Input: part model. Units: mm. Frame: model coordinates. Face numbers are marked on the shaded views. Coordinates: 2 decimals unless noted, no trailing zeros. Order: outer loops, then holes, each group sorted by start corner. A loop starts at its lowest first (then second) coordinate and runs counter-clockwise, first axis right, second up. Notation, with made-up numbers: M 51.25,80.25 L 83.25,80.25 A17 ccw 83.25,106.25 Z; hole C -39.5,-13 d3. An arc over 180 degrees is marked long. One line per item, written item: value.
```python
from build123d import *

# Parameters (mm, degrees)
SKETCH1_W           = 23.075946232
SKETCH1_H           = 15.72
SKETCH1_R           = 1.525
SKETCH1_R_2         = 4.5
BOSS_EXTRUDE2_DEPTH = 4


with BuildPart() as part:
    # Sketch1 → Boss-Extrude2 (new body)
    with BuildSketch(Plane.XY):
        Rectangle(SKETCH1_W, SKETCH1_H)
        with Locations((-8.105997779, -4.68)):
            Circle(SKETCH1_R, mode=Mode.SUBTRACT)
        with Locations((8.105997779, -4.68)):
            Circle(SKETCH1_R, mode=Mode.SUBTRACT)
        with Locations((8.105997779, 4.68)):
            Circle(SKETCH1_R, mode=Mode.SUBTRACT)
        with Locations((-8.105997779, 4.68)):
            Circle(SKETCH1_R, mode=Mode.SUBTRACT)
        Polygon((3.671947712, -6.36), (7.343895424, 0), (3.671947712, 6.36), (-3.671947712, 6.36), (-7.343895424, 0), (-3.671947712, -6.36), align=None, mode=Mode.SUBTRACT)
        Polygon((-3.671947712, -6.36), (3.671947712, -6.36), (7.343895424, 0), (3.671947712, 6.36), (-3.671947712, 6.36), (-7.343895424, 0), align=None)
        Circle(SKETCH1_R_2, mode=Mode.SUBTRACT)
    extrude(amount=BOSS_EXTRUDE2_DEPTH)


solid = part.part
```
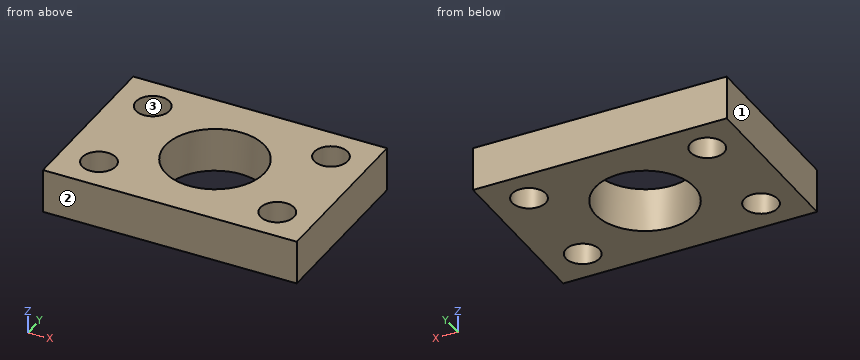
(1) Cut plane C-C on y = 0. Output: boundary loops of the cut face in (x, z).
Data:
outline: M -11.54,0 L -4.5,0 L -4.5,4 L -11.54,4 Z; M 4.5,0 L 11.54,0 L 11.54,4 L 4.5,4 Z
(2) Cut plane A-A on x = 0. Output: boundary loops of the cut face in (y, z).
Data:
outline: M -7.86,0 L -4.5,0 L -4.5,4 L -7.86,4 Z; M 4.5,0 L 7.86,0 L 7.86,4 L 4.5,4 Z
(3) Ray query, line 1 (Y direction, x = -8, z = 0.75); line 2 (X direction, y = 5, z = 0.2); line 3 (Y direction, x = -3.25, z = 3.05). Return the intervals inside material, ascending. Write a range as from..to.
Data:
line 1: y = -7.86..-6.2, -3.16..3.16, 6.2..7.86
line 2: x = -11.54..-9.6, -6.61..6.61, 9.6..11.54
line 3: y = -7.86..-3.11, 3.11..7.86
(4) First-contact query: pin 1 (4 mm diameter, centred on x = -8.11, y = 4.68, fed in from +Z). Flat tip, straight axial feed; report the tip coordinate or a pass-through.
Data:
pin 1: stops at z = 4
(5) Cut plane B-B on z = 3.7. Output: boundary loops of the cut face in (x, y) (3 decimals), plus the area to 3 significant figures.
Data:
outline: M -11.538,-7.86 L 11.538,-7.86 L 11.538,7.86 L -11.538,7.86 Z; hole C -8.106,-4.68 d3.05; hole C -8.106,4.68 d3.05; hole C 0,0 d9; hole C 8.106,-4.68 d3.05; hole C 8.106,4.68 d3.05
area: 270 mm2
(6) Draft query along Y for the marked faces 1, 2 and 3. Return one class per face: released by +Y, released by -Y, zero draft, split by the parting line, or undercut.
Data:
face 1: zero draft
face 2: released by -Y
face 3: undercut
(7) Cut plane D-D on x = 8. Output: boundary loops of the cut face in (y, z).
Data:
outline: M -7.86,0 L -6.2,0 L -6.2,4 L -7.86,4 Z; M -3.16,0 L 3.16,0 L 3.16,4 L -3.16,4 Z; M 6.2,0 L 7.86,0 L 7.86,4 L 6.2,4 Z
